Build history of the part. All positions in model axes, mm. Round coordinates to 2 decimals unless told otherwise and drop trailing zeros. Write each loop counter-clockwise with the first axis right and the second up, starting at its lowest first coordinate (ties: lowest second). Pieces come first, ordered by that corner, then holes. Notation, with made-up numbers: (-11.5, 35.5) -> (16.5, 35.5) arc R8 cw to (16.5, 44.5) -> close; hole circle Ø5 at (-28.5, -23). An arc over 180 degrees is marked (long way). Answer as CSV lines item,"result".
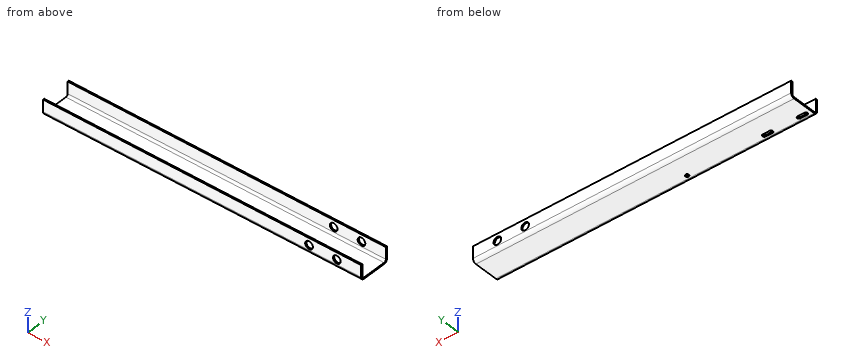
from build123d import *

# Parameters (mm, degrees)
SKETCH1_W                    = 915
SKETCH1_H                    = 88
BASE_FLANGE1_DEPTH           = 4
EDGE_FLANGE1_STRIP_W         = 28
EDGE_FLANGE1_STRIP_H         = 4
EDGE_FLANGE1_STRIP_CUT_DEPTH = 915
EDGE_FLANGE1_DEPTH           = 915
EDGE_FLANGE2_STRIP_W         = 28
EDGE_FLANGE2_STRIP_H         = 4
EDGE_FLANGE2_STRIP_CUT_DEPTH = 915
EDGE_FLANGE2_DEPTH           = 915
CUT_EXTRUDE1_DEPTH           = 871.900176512
CUT_EXTRUDE1_DEPTH_BACK      = 871.900176512
SKETCH12_R                   = 11
CUT_EXTRUDE2_DEPTH           = 872.093059006
SKETCH16_R                   = 5
CUT_EXTRUDE4_DEPTH           = 10


# Sheet-metal steps are written as plain solids
with BuildPart() as part:
    # Sketch1 → Base-Flange1 (new body)
    with BuildSketch(Plane.XY):
        with Locations((-408.018987342, 44)):
            Rectangle(SKETCH1_W, SKETCH1_H)
    extrude(amount=-BASE_FLANGE1_DEPTH)

    # Edge-Flange1 strip (across the edge) → Edge-Flange1 strip cut (cut)
    with BuildSketch(Plane(origin=(49.481012658, 88, 0), x_dir=(0, -1, 0), z_dir=(-1, 0, 0))):
        with Locations((-4, -2)):
            Rectangle(EDGE_FLANGE1_STRIP_W, EDGE_FLANGE1_STRIP_H)
    extrude(amount=EDGE_FLANGE1_STRIP_CUT_DEPTH, mode=Mode.SUBTRACT)

    # Edge-Flange1 section (across the edge) → Edge-Flange1 (add)
    with BuildSketch(Plane(origin=(49.481012658, 88, 0), x_dir=(0, -1, 0), z_dir=(-1, 0, 0))):
        with BuildLine():
            Line((0, 6), (0, 40))
            Line((0, 40), (4, 40))
            Line((4, 40), (4, 6))
            ThreePointArc((4, 6), (5.757359313, 1.757359313), (10, 0))
            Line((10, 0), (10, -4))
            ThreePointArc((10, -4), (2.928932188, -1.071067812), (0, 6))
        make_face()
    extrude(amount=EDGE_FLANGE1_DEPTH)

    # Edge-Flange2 strip (across the edge) → Edge-Flange2 strip cut (cut)
    with BuildSketch(Plane.YZ.offset(-865.518987342)):
        with Locations((-4, -2)):
            Rectangle(EDGE_FLANGE2_STRIP_W, EDGE_FLANGE2_STRIP_H)
    extrude(amount=EDGE_FLANGE2_STRIP_CUT_DEPTH, mode=Mode.SUBTRACT)

    # Edge-Flange2 section (across the edge) → Edge-Flange2 (add)
    with BuildSketch(Plane.YZ.offset(-865.518987342)):
        with BuildLine():
            Line((0, 6), (0, 40))
            Line((0, 40), (4, 40))
            Line((4, 40), (4, 6))
            ThreePointArc((4, 6), (5.757359313, 1.757359313), (10, 0))
            Line((10, 0), (10, -4))
            ThreePointArc((10, -4), (2.928932188, -1.071067812), (0, 6))
        make_face()
    extrude(amount=EDGE_FLANGE2_DEPTH)

    # Sketch12 → Cut-Extrude1 (cut, two sides: drawn at the far end of the back side and taken through both)
    with BuildSketch(Plane.XZ.offset(-CUT_EXTRUDE1_DEPTH_BACK)):
        with Locations(Location((-100.518987342, 20, 0), (0, 0, 270))):
            Circle(SKETCH12_R)
        with Locations(Location((-20.518987342, 20, 0), (0, 0, 270))):
            Circle(SKETCH12_R)
    extrude(amount=CUT_EXTRUDE1_DEPTH + CUT_EXTRUDE1_DEPTH_BACK, mode=Mode.SUBTRACT)

    # Sketch13 → Cut-Extrude2 (cut, through all)
    with BuildSketch(Plane(origin=(0, 0, -4), x_dir=(-1, 0, 0), z_dir=(0, 0, -1))):
        with BuildLine():
            Line((850.518987342, 15), (830.518987342, 15))
            ThreePointArc((830.518987342, 15), (825.518987342, 20), (830.518987342, 25))
            Line((830.518987342, 25), (850.518987342, 25))
            ThreePointArc((850.518987342, 25), (855.518987342, 20), (850.518987342, 15))
        make_face()
        with BuildLine():
            Line((750.518987342, 15), (730.518987342, 15))
            ThreePointArc((730.518987342, 15), (725.518987342, 20), (730.518987342, 25))
            Line((730.518987342, 25), (750.518987342, 25))
            ThreePointArc((750.518987342, 25), (755.518987342, 20), (750.518987342, 15))
        make_face()
    extrude(amount=-CUT_EXTRUDE2_DEPTH, mode=Mode.SUBTRACT)

    # Sketch16 → Cut-Extrude4 (cut)
    with BuildSketch(Plane(origin=(0, 0, -4), x_dir=(-1, 0, 0), z_dir=(0, 0, -1))):
        with Locations((509.018987342, 20)):
            Circle(SKETCH16_R)
    extrude(amount=-CUT_EXTRUDE4_DEPTH, mode=Mode.SUBTRACT)


solid = part.part
1. Cut at B-B, the plane x = -303.5. Write the cut outline in (y, z), then the cut area to 3 significant figures.
Results found:
outline,"(0, 6) arc R10 ccw to (10, -4) -> (78, -4) arc R10 ccw to (88, 6) -> (88, 40) -> (84, 40) -> (84, 6) arc R6 cw to (78, 0) -> (10, 0) arc R6 cw to (4, 6) -> (4, 40) -> (0, 40) -> close"
area,"645 mm2"
2. Cut at A-A, the plane z = 20. Write the cut outline in (x, y), then the cut area to 3 significant figures.
Results found:
outline,"(-865.52, 0) -> (-111.52, 0) -> (-111.52, 4) -> (-865.52, 4) -> close; (-865.52, 84) -> (-111.52, 84) -> (-111.52, 88) -> (-865.52, 88) -> close; (-89.52, 0) -> (-31.52, 0) -> (-31.52, 4) -> (-89.52, 4) -> close; (-89.52, 84) -> (-31.52, 84) -> (-31.52, 88) -> (-89.52, 88) -> close; (-9.52, 0) -> (49.48, 0) -> (49.48, 4) -> (-9.52, 4) -> close; (-9.52, 84) -> (49.48, 84) -> (49.48, 88) -> (-9.52, 88) -> close"
area,"6,970 mm2"
3. Drop flat-ended pins along their axis: pin 1 Ø3 at (x, z) = (-845.5, -1.5) entering from +Y; pin 2 Ø2 at (x, z) = (-837.5, -2) entering from -Y; pin 3 Ø4.5 at (x, z) = (-740.5, -2.5) entering from +Y. Give the stop position or say it passes through.
Results found:
pin 1,"stops at y = 86"
pin 2,"stops at y = 2.86"
pin 3,"stops at y = 85.81"
4. Cut at C-C, the plane y = 58. Write the cut outline in (x, z).
Results found:
outline,"(-865.52, -4) -> (49.48, -4) -> (49.48, 0) -> (-865.52, 0) -> close"
5. Probe line 1 along X through (y, z) = (86.2, 20); line 2 along Y through (x, z) = (-694, 14.5); line 3 along Z through (x, y) = (-803.5, 11.5). List the from-to ranges inside material, lowest first.
Results found:
line 1,"x = -865.52 to -111.52, -89.52 to -31.52, -9.52 to 49.48"
line 2,"y = 0 to 4, 84 to 88"
line 3,"z = -4 to 0"
